Autodesk Inventor part; units mm, degrees
ref_plane "YZ Plane" through (0, 0, 0) normal (1, 0, 0) x (0, 1, 0)
ref_plane "XZ Plane" through (0, 0, 0) normal (0, 1, 0) x (-1, 0, 0)
ref_plane "XY Plane" through (0, 0, 0) normal (0, 0, 1) x (1, 0, 0)
sketch "Sketch1" plane through (38.1, 172.72, 38.1) normal (0, 1, 0) x (-1, 0, 0)
  line L0 (38.1, 773.5975) -> (-850.9, 773.5975)
  line L1 (38.1, 773.5975) -> (165.1, 773.5975)
  line L2 (165.1, 773.5975) -> (165.1, -38.1)
  line L3 (165.1, -38.1) -> (165.1, -241.3)
  line L4 (165.1, -241.3) -> (-850.9, -241.3)
  line L5 (-850.9, -241.3) -> (-850.9, 773.5975)
  line L6 (165.1, -241.3) -> (165.1, -292.1)
  line L7 (165.1, -292.1) -> (-850.9, -292.1)
  line L8 (-850.9, -292.1) -> (-850.9, -241.3)
  point P0 (38.1, -38.1)
  dimension "d0" = 889
  dimension "d1" = 127
  dimension "d2" = 203.2
  dimension "d3" = 1014.8975
  dimension "d4" = 811.6975
  dimension "d9" = 50.8
sketch "Sketch2" plane through (0, 15.24, 0) normal (0, 0, -1) x (-1, 0, 0)
  line L0 (-309.1034, 107.227) -> (-309.1034, 38.647)
  line L1 (-272.9596, 74.2658) -> (-488.8596, 74.2658)
  line L2 (-272.9596, 38.647) -> (-488.8596, 38.647)
  line L3 (-488.8596, 38.647) -> (-488.8596, 107.227)
  line L4 (-488.8596, 107.227) -> (-272.9596, 107.227)
  line L5 (-272.9596, 107.227) -> (-272.9596, 38.647)
  point P0 (0, -15.24)
  dimension "d5" = 215.9
  dimension "d6" = 68.58
ref_plane "Work Plane1" through (272.9596, 122.4669, 0) normal (0, 1, 0) x (1, 0, 0)
sketch "Sketch3" plane through (272.9596, 122.4669, 0) normal (0, 1, 0) x (1, 0, 0)
  point P0 (-272.9596, 0)
extrude "Extrusion2" add sketch "Sketch1" along normal blind 101.6
sketch "Sketch4" plane through (38.1, 172.72, 38.1) normal (0, -1, 0) x (1, 0, 0)
  line L0 (-165.1, -292.1) -> (-165.1, 773.5975)
  line L1 (-165.1, -292.1) -> (-165.1, 773.5975)
  line L2 (-165.1, 773.5975) -> (-38.1, 773.5975)
  line L3 (-165.1, 773.5975) -> (850.9, 773.5975)
  line L4 (-38.1, -38.1) -> (-38.1, 773.5975)
  line L5 (-38.1, -38.1) -> (723.083, -38.1)
  line L6 (723.083, -38.1) -> (723.083, 773.5975)
  line L7 (723.083, 773.5975) -> (850.9, 773.5975)
  line L8 (850.9, 773.5975) -> (850.9, -292.1)
  line L9 (850.9, 773.5975) -> (850.9, -292.1)
  line L10 (850.9, -292.1) -> (-165.1, -292.1)
  line L11 (850.9, -292.1) -> (-165.1, -292.1)
extrude "Extrusion3" add sketch "Sketch4" along normal blind 172.72 contours L0 L2 L4 L5 L6 L3 L8 L10
extrude "Extrusion4" cut sketch "Sketch2" along normal blind 203.2
sketch "Sketch5" plane through (761.183, 172.72, 0) normal (-1, 0, 0) x (0, 0, 1)
  line L0 (0, -172.72) -> (811.6975, -172.72)
  line L1 (0, 0) -> (0, -172.72)
  line L2 (811.6975, -172.72) -> (0, -172.72)
  line L3 (0, -172.72) -> (0, 0)
  line L4 (0, 0) -> (811.6975, 0)
  line L5 (811.6975, 0) -> (811.6975, -172.72)
  point P0 (0, -172.72)
extrude "Extrusion5" cut sketch "Sketch5" against normal blind 2.54
sketch "Sketch6" plane through (0, 172.72, 811.6975) normal (1, 0, 0) x (0, 0, -1)
  line L0 (0, -172.72) -> (1065.6975, -172.72)
  line L1 (0, 0) -> (811.6975, 0)
  line L2 (0, -172.72) -> (811.6975, -172.72)
  line L3 (811.6975, -172.72) -> (811.6975, 0)
  line L4 (811.6975, 0) -> (0, 0)
  line L5 (0, 0) -> (0, -172.72)
  point P0 (811.6975, -172.72)
extrude "Extrusion6" cut sketch "Sketch6" against normal blind 2.54
properties part number "ExpansionCard1"
Read the model definition and answer for the solid it produces. Units are mm, in the model's axes. A direction names the side the tool comes from. Round coordinates to 2 decimals unless told otherwise and drop trailing zeros. Write each loop counter-clockwise with the first axis right and the second up, starting at its lowest first coordinate (ties: lowest second). Pieces come first, ordered by that corner, then holes.
Q1. Find section D-D on x = 325.5. Determine the outline of the cut face in (y, z), and give its area (3 significant figures).
Values:
outline: (0, -254) - (274.32, -254) - (274.32, 811.7) - (172.72, 811.7) - (172.72, 0) - (122.47, 0) - (122.47, -203.2) - (53.89, -203.2) - (53.89, 0) - (0, 0) - close
area: 138,000 mm2
Q2. Find section B-B on y = 73.5. Determine the outline of the cut face in (x, z), and give its area (3 significant figures).
Values:
outline: (-127, -254) - (889, -254) - (889, 811.7) - (763.72, 811.7) - (763.72, 0) - (488.86, 0) - (488.86, -203.2) - (272.96, -203.2) - (272.96, 0) - (-2.54, 0) - (-2.54, 811.7) - (-127, 811.7) - close
area: 417,000 mm2
Q3. Find section C-C on z = 290.5. Determine the outline of the cut face in (x, y).
Values:
outline: (-127, 0) - (-2.54, 0) - (-2.54, 172.72) - (763.72, 172.72) - (763.72, 0) - (889, 0) - (889, 274.32) - (-127, 274.32) - close
Q4. A tool of negligible diameter and unlimited length cuts with its end or side. For faces 1 (the face through (-2.54, 88, 412)), 2 (the face through (388, 139, -254)), 3 (the face through (272.96, 89, -100)), from which of +Z, -Z, +X, -X, +Y, -Y can it reach the whole face along a straight path? Write none if from no direction.
Values:
face 1: +Z, -Y
face 2: -Z, +X, -X, +Y, -Y
face 3: +Z
Q5. A flat-ended cylindrical pin translates along its axis: P1, Ø8, axis at x = 62.5, y = 100.5, coming from the +Z side. Find the tip coordinate at first contact, or state that the pin passes through.
Values:
P1: stops at z = 0
Q6. Straight lines are drawn through the part: line 1 (X direction, y = 150, z = 279.5); line 2 (Y direction, x = 354, z = -168); line 3 (Y direction, x = 539.5, z = 95). For each, find the intervals that lie inside material, in ascending order.
Values:
line 1: x = -127 to -2.54, 763.72 to 889
line 2: y = 0 to 53.89, 122.47 to 274.32
line 3: y = 172.72 to 274.32
Q7. The mould has two halves that part along Y. Classify faces 4 (the face through (382, 89, -203.2)), 5 (the face through (488.86, 88, -100)), 6 (the face through (388, 274.32, 286)), 7 (the face through (375, 172.72, 400)): released by +Y, released by -Y, zero draft, split by the parting line, or undercut.
Values:
face 4: undercut
face 5: undercut
face 6: released by +Y
face 7: released by -Y
Q8. Find section A-A on z = -99.5. Determine the outline of the cut face in (x, y), and give its area (3 significant figures).
Values:
outline: (-127, 0) - (889, 0) - (889, 274.32) - (-127, 274.32) - close; hole (272.96, 53.89) - (488.86, 53.89) - (488.86, 122.47) - (272.96, 122.47) - close
area: 264,000 mm2
